```python
from build123d import *

# Parameters (mm, degrees)
CROQUIS1_W              = 65
CROQUIS1_H              = 100
SALIENTE_EXTRUIR1_DEPTH = 50
REDONDEO1_R             = 10
VACIADO1_START          = 5
VACIADO1_DEPTH          = 90
CROQUIS3_R              = 6
CORTAR_EXTRUIR1_DEPTH   = 130.325171564


# Read off the part's stored shape, not the designer's step: Vaciado1
with BuildPart() as part:
    # Croquis1 → Saliente-Extruir1 (new body)
    with BuildSketch(Plane(origin=(0, 0, 0), x_dir=(0, 0, -1), z_dir=(1, 0, 0))):
        with Locations((32.5, 50)):
            Rectangle(CROQUIS1_W, CROQUIS1_H)
    extrude(amount=SALIENTE_EXTRUIR1_DEPTH)

    # Redondeo1
    redondeo1_edges = [part.edges().sort_by_distance(p)[0] for p in [
        (50, 50, -65),
        (50, 50, 0),
        (0, 50, -65),
        (0, 50, 0),
    ]]
    fillet(redondeo1_edges, radius=REDONDEO1_R)

    # Vaciado1 outline → Vaciado1 (cut)
    with BuildSketch(Plane(origin=(0, 0, 0), x_dir=(1, 0, 0), z_dir=(0, 1, 0)).offset(VACIADO1_START)):
        with BuildLine():
            Line((10, 0), (40, 0))
            Line((40, 0), (40, 5))
            ThreePointArc((40, 5), (43.535533906, 6.464466094), (45, 10))
            Line((45, 10), (45, 55))
            ThreePointArc((45, 55), (43.535533906, 58.535533906), (40, 60))
            Line((40, 60), (10, 60))
            ThreePointArc((10, 60), (6.464466094, 58.535533906), (5, 55))
            Line((5, 55), (5, 10))
            ThreePointArc((5, 10), (6.464466094, 6.464466094), (10, 5))
            Line((10, 5), (10, 0))
        make_face()
    extrude(amount=VACIADO1_DEPTH, mode=Mode.SUBTRACT)

    # Croquis3 → Cortar-Extruir1 (cut, through all)
    with BuildSketch(Plane(origin=(0, 100, 0), x_dir=(1, 0, 0), z_dir=(0, 1, 0))):
        with Locations(Location((25.623850115, 30, 0), (0, 0, 270))):
            Circle(CROQUIS3_R)
    extrude(amount=-CORTAR_EXTRUIR1_DEPTH, mode=Mode.SUBTRACT)


solid = part.part
```
The listing builds one solid part. Answer for the finished solid, in the listing's coordinates (mm). A direction names the side the tool comes from. Round coordinates to 2 decimals unless told otherwise and drop trailing zeros. Order: outer loops, then holes, each group sorted by start corner. A loop starts at its lowest first (then second) coordinate and runs counter-clockwise, first axis right, second up. Notation, with made-up numbers: (1.25, 75) - (41.25, 75) arc R26 cw to (41.25, 93) - close; hole circle Ø3 at (-30, -15.75). An arc over 180 degrees is marked (long way). Put each result on its own line as item: value. Start each with the question number.
(1) Find section D-D (x = 22). Give the vertices of the cut face in (y, z).
(2) Given P1, Ø4, axis at y = 62, z = -2.5, coming from the -X side; P2, Ø15, axis at x = 31.5, y = 50, coming from the +Z side; P3, Ø5.5, axis at y = 63.5, z = -3, coming from the +X side, each flat-ended and moving along its own axis, determine where each tip first touches the part or whether it passes through.
(3) Find section B-B (z = -30). Give the vertices of the cut face in (x, y), plus the area to 3 significant figures.
(4) Straight lines are drawn through the part: probe 1 along X at (y, z) = (51, -27); probe 2 along X at (y, z) = (1.4, -30); probe 3 along Y at (x, z) = (23.5, -54.5). For each, find the intervals that lie inside material, in ascending order. Write a range as from..to.
(5) Find section C-C (y = 73.5). Give the vertices of the cut face in (x, z).
(6) Find section A-A (z = -48.5). Give the vertices of the cut face in (x, y).
(7) For faces 1 (the cylindrical face through (6, 49, -7)), 2 (the flat face through (40, 49, -2)), 3 (the flat face through (25, 2, 0)), determine the directions among +Z, -Z, +X, -X, +Y, -Y from which every point of the face is accessible in a straight line to the end or side of a thin tool.
(8) Determine the mould class of faces 4 (the flat face through (10, 49, -3)), 5 (the flat face through (25, 49, -65)), 6 (the flat face through (19, 100, -32)) for opening direction Y: released by +Y, released by -Y, zero draft, split by the parting line, or undercut.
Reply:
1. outline: (0, -65) - (100, -65) - (100, -34.78) - (95, -34.78) - (95, -60) - (5, -60) - (5, -34.78) - (0, -34.78) - close; (0, -25.22) - (5, -25.22) - (5, 0) - (0, 0) - close; (95, -25.22) - (100, -25.22) - (100, 0) - (95, 0) - close
2. P1: x = 1.65
2. P2: z = -60
2. P3: x = 49.05
3. outline: (0, 0) - (19.62, 0) - (19.62, 5) - (5, 5) - (5, 95) - (19.62, 95) - (19.62, 100) - (0, 100) - close; (31.62, 0) - (50, 0) - (50, 100) - (31.62, 100) - (31.62, 95) - (45, 95) - (45, 5) - (31.62, 5) - close
3. area: 1,280 mm^2
4. probe 1: 0..5, 45..50
4. probe 2: 0..19.62, 31.62..50
4. probe 3: 0..5, 95..100
5. outline: (0, -55) arc R10 ccw to (10, -65) - (40, -65) arc R10 ccw to (50, -55) - (50, -10) arc R10 ccw to (40, 0) - (40, -5) arc R5 cw to (45, -10) - (45, -55) arc R5 cw to (40, -60) - (10, -60) arc R5 cw to (5, -55) - (5, -10) arc R5 cw to (10, -5) - (10, 0) arc R10 ccw to (0, -10) - close
6. outline: (0, 0) - (50, 0) - (50, 100) - (0, 100) - close; hole (5, 5) - (45, 5) - (45, 95) - (5, 95) - close
7. face 1: none
7. face 2: +Z
7. face 3: +Z, +X, -X, +Y, -Y
8. face 4: undercut
8. face 5: zero draft
8. face 6: released by +Y
